Answer from the drawing. Dimensions are ordinates in mm from the lowest x, y and z of the part. Give positions to 0.01 mm unless a question says otherwise; leave off trailing zeros. Order: outer loops, then holes, each group sorted by start corner. A loop starts at its lowest first (then second) coordinate and runs counter-clockwise, first axis right, second up. Notation, with made-up numbers: (-3, 12) - (2, 12) arc R7 ccw to (2, 22) - close; hole circle Ø6 at (25.25, -18.5). An arc over 180 degrees is marked (long way). Write each question's results on one line, items separated by ' | '.
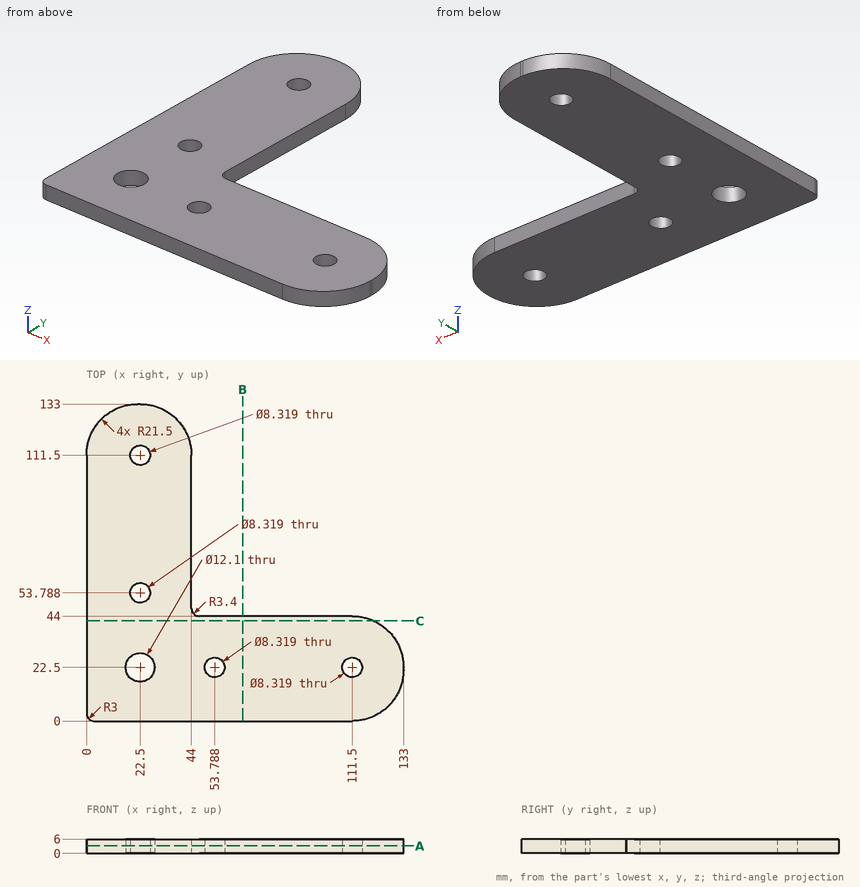
1. A cutting plane is placed at B-B, the plane x = 65.5. Write down the section's boundary in (y, z).
Answer list:
outline: (0, 0) - (44, 0) - (44, 6) - (0, 6) - close
2. Straight lines are drawn through the part: line 1 (Y direction, x = 111.5, z = 2.6); line 2 (Y direction, x = 69.5, z = 4.05). For each, find the intervals that lie inside material, in ascending order. Write a range as [from, to].
Answer list:
line 1: [0, 18.34], [26.66, 44] | line 2: [0, 44]
3. Given P1, Ø3, axis at y = 86, z = 3, coming from the +X side; P2, Ø1, axis at y = 19, z = 3, coming from the +X side, each flat-ended and moving along its own axis, determine where each tip first touches the part or whether it passes through.
Answer list:
P1: x = 44 | P2: x = 132.91
4. A cutting plane is placed at A-A, the plane z = 3.15. Write down the section's boundary in (x, y), then the cut area to 3 significant figures.
Answer list:
outline: (0, 3) arc R3 ccw to (3, 0) - (111.5, 0) arc R21.5 ccw to (133, 21.5) - (133, 22.5) arc R21.5 ccw to (111.5, 44) - (47.4, 44) arc R3.4 cw to (44, 47.4) - (44, 111.5) arc R21.5 ccw to (22.5, 133) - (21.5, 133) arc R21.5 ccw to (0, 111.5) - close; hole circle Ø12.1 at (22.5, 22.5); hole circle Ø8.32 at (22.5, 53.79); hole circle Ø8.32 at (22.5, 111.5); hole circle Ø8.32 at (53.79, 22.5); hole circle Ø8.32 at (111.5, 22.5) | area: 9,040 mm^2
5. A cutting plane is placed at C-C, the plane y = 42. Write down the section's boundary in (x, z) (1 decimal).
Answer list:
outline: (0, 0) - (120.6, 0) - (120.6, 6) - (0, 6) - close
